Check sheet for the modelled part. Datum: model origin and axes. Units: mm. A direction names the side the tool comes from. Round coordinates to 2 decimals unless told otherwise and drop trailing zeros. Order: outer loops, then holes, each group sorted by start corner. A loop starts at its lowest first (then second) coordinate and runs counter-clockwise, first axis right, second up.
```python
from build123d import *

# Parameters (mm, degrees)
F0_W      = 1143
F0_H      = 355.6
F0_W_2    = 838.2
F0_H_2    = 342.9
F1_DEPTH  = 50.8
F2_W      = 139.7
F2_H      = 342.9
F3_DEPTH  = 44.45
F4_W      = 1143
F4_H      = 3.175
F5_DEPTH  = 25.4
F6_W      = 1143
F6_H      = 3.175
F7_DEPTH  = 25.4
F9_DEPTH  = 50.8
F10_SIZE  = 50.8
F13_DEPTH = 571.5
F14_SIZE  = 2.54


with BuildPart() as f1:
    # F0 (on Top) → F1 (new body)
    with BuildSketch(Plane.XY):
        Rectangle(F0_W, F0_H)
        Rectangle(F0_W_2, F0_H_2, mode=Mode.SUBTRACT)
    extrude(amount=F1_DEPTH)

    # F2 (on face) → F3 (cut)
    with BuildSketch(Plane.XY.offset(50.8)):
        with Locations((-495.3, 0)):
            Rectangle(F2_W, F2_H)
        with Locations((495.3, 0)):
            Rectangle(F2_W, F2_H)
    extrude(amount=-F3_DEPTH, mode=Mode.SUBTRACT)

    # F4 (on face) → F5 (join)
    with BuildSketch(Plane(origin=(0, 177.8, 0), x_dir=(-1, 0, 0), z_dir=(0, 1, 0))):
        with Locations((0, 49.2125)):
            Rectangle(F4_W, F4_H)
    extrude(amount=F5_DEPTH)

    # F6 (on face) → F7 (join)
    with BuildSketch(Plane.XZ.offset(177.8)):
        with Locations((0, 49.2125)):
            Rectangle(F6_W, F6_H)
    extrude(amount=F7_DEPTH)

    # F8 (on face) → F9 (join)
    with BuildSketch(Plane(origin=(0, 0, 0), x_dir=(1, 0, 0), z_dir=(0, 0, -1))):
        Polygon((-419.1, 177.8), (-571.5, 177.8), (-571.5, -177.8), (-419.1, -177.8), (-419.1, -171.45), (-419.1, 171.45), align=None)
        Polygon((571.5, 177.8), (419.1, 177.8), (419.1, 171.45), (419.1, -171.45), (419.1, -177.8), (571.5, -177.8), align=None)
    extrude(amount=F9_DEPTH)

    # F10
    f10_edges = [f1.edges().sort_by_distance(p)[0] for p in [
        (-495.3, 177.8, -50.8),
        (-495.3, -177.8, -50.8),
        (495.3, -177.8, -50.8),
        (495.3, 177.8, -50.8),
    ]]
    chamfer(f10_edges, length=F10_SIZE)

    # F11 (on face) + F12 (on face) → F13 (join)
    with BuildSketch(Plane(origin=(0, 0, -50.8), x_dir=(1, 0, 0), z_dir=(0, 0, -1))):
        Polygon((457.2, -63.5), (495.3, -63.5), (533.4, -63.5), (533.4, 63.5), (457.2, 63.5), align=None)
        Polygon((527.05, -57.15), (495.3, -57.15), (463.55, -57.15), (463.55, 57.15), (527.05, 57.15), align=None, mode=Mode.SUBTRACT)
    with BuildSketch(Plane(origin=(0, 0, -50.8), x_dir=(1, 0, 0), z_dir=(0, 0, -1))):
        Polygon((-533.4, -63.5), (-495.3, -63.5), (-457.2, -63.5), (-457.2, 63.5), (-533.4, 63.5), align=None)
        Polygon((-463.55, -57.15), (-495.3, -57.15), (-527.05, -57.15), (-527.05, 57.15), (-463.55, 57.15), align=None, mode=Mode.SUBTRACT)
    extrude(amount=F13_DEPTH)

    # F14
    f14_edges = [f1.edges().sort_by_distance(p)[0] for p in [
        (-457.2, -63.5, -336.55),
        (-533.4, -63.5, -336.55),
        (-457.2, 63.5, -336.55),
        (533.4, -63.5, -336.55),
        (457.2, -63.5, -336.55),
        (533.4, 63.5, -336.55),
        (457.2, 63.5, -336.55),
        (-533.4, 63.5, -336.55),
    ]]
    chamfer(f14_edges, length=F14_SIZE)


solid = f1.part
```
Item 1: Sectioned sample at C-C (x = 92.5). Record the cut outline in (y, z) (3 decimals), and give its area (3 significant figures).
Answer:
outline: (-203.2, 47.625) - (-177.8, 47.625) - (-177.8, 0) - (-171.45, 0) - (-171.45, 50.8) - (-203.2, 50.8) - close; (171.45, 0) - (177.8, 0) - (177.8, 47.625) - (203.2, 47.625) - (203.2, 50.8) - (171.45, 50.8) - close
area: 806 mm2
Item 2: Go/stop test with flat-tipped pins: P1, Ø8, axis at y = 38, z = -329, coming from the +X side; P2, Ø3, axis at x = -84, y = 174, coming from the -Z side; P3, Ø13.5, axis at x = -473.5, z = 28, coming from the +Y side. Record where each tip stops, or that it passes through.
Answer:
P1: stops at x = 533.4
P2: stops at z = 0
P3: stops at y = 177.8
Item 3: Scan lines: line 1 along X through (y, z) = (-43.5, -258.5); line 2 along Y through (x, z) = (346.5, 19); line 3 along X through (y, z) = (-59, -593). Record each from-to range of solid material in increasing order.
Answer:
line 1: x = -533.4 to -527.05, -463.55 to -457.2, 457.2 to 463.55, 527.05 to 533.4
line 2: y = -177.8 to -171.45, 171.45 to 177.8
line 3: x = -533.4 to -457.2, 457.2 to 533.4
Item 4: Access from +Z, -Z, +X, -X, +Y, -Y to the whole of each face (thin tool, end or side, straight path). Record for faces 1 (the flat face through (425.45, -2, 29)), 2 (the flat face through (8, 190, 47.625)), 3 (the flat face through (463.55, 1, -333)).
Answer:
face 1: +Z
face 2: -Z, +X, -X, +Y
face 3: -Z
Item 5: Release check for a two-part mould opening along Y. For faces 4 (the flat face through (495, -1, -50.8)), 5 (the flat face through (-495, -63.5, -333)), 6 (the flat face through (545, -2, -50.8)) record: released by +Y, released by -Y, zero draft, split by the parting line, or undercut.
Answer:
face 4: undercut
face 5: released by -Y
face 6: zero draft
Item 6: Sectioned sample at B-B (y = -91.5). Record the cut outline in (x, z).
Answer:
outline: (-571.5, -50.8) - (-419.1, -50.8) - (-419.1, 50.8) - (-425.45, 50.8) - (-425.45, 6.35) - (-565.15, 6.35) - (-565.15, 50.8) - (-571.5, 50.8) - close; (419.1, -50.8) - (571.5, -50.8) - (571.5, 50.8) - (565.15, 50.8) - (565.15, 6.35) - (425.45, 6.35) - (425.45, 50.8) - (419.1, 50.8) - close
Item 7: Sectioned sample at A-A (z = -246). Record the cut outline in (x, y).
Answer:
outline: (-533.4, -60.96) - (-530.86, -63.5) - (-459.74, -63.5) - (-457.2, -60.96) - (-457.2, 60.96) - (-459.74, 63.5) - (-530.86, 63.5) - (-533.4, 60.96) - close; (457.2, -60.96) - (459.74, -63.5) - (530.86, -63.5) - (533.4, -60.96) - (533.4, 60.96) - (530.86, 63.5) - (459.74, 63.5) - (457.2, 60.96) - close; hole (-527.05, -57.15) - (-463.55, -57.15) - (-463.55, 57.15) - (-527.05, 57.15) - close; hole (463.55, -57.15) - (527.05, -57.15) - (527.05, 57.15) - (463.55, 57.15) - close
